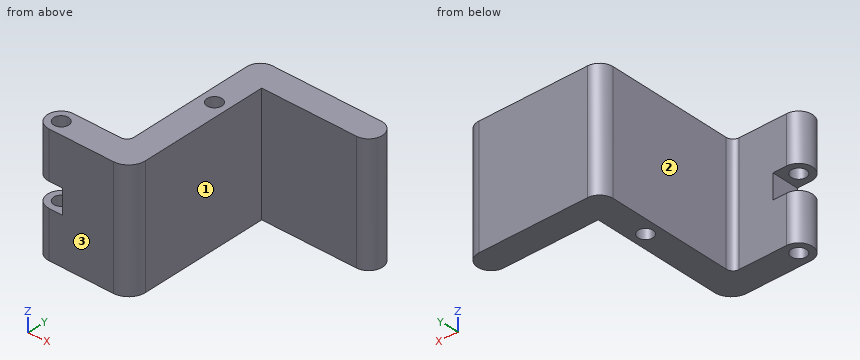
from build123d import *

# Parameters (mm, degrees)
BOSS_EXTRUDE1_DEPTH     = 87.5
SKETCH2_R               = 11
CUT_EXTRUDE1_DEPTH      = 175
FILLET1_R               = 10
FILLET2_R               = 25
CUT_EXTRUDE2_DEPTH      = 18
CUT_EXTRUDE2_DEPTH_BACK = 18
SKETCH3_W               = 40
SKETCH3_H               = 40
BOSS_EXTRUDE2_START     = -175
BOSS_EXTRUDE2_DEPTH     = 175


with BuildPart() as part:
    # Sketch1 → Boss-Extrude1 (new, symmetric)
    with BuildSketch(Plane.XY):
        with BuildLine():
            Line((-20, 20), (-20, 140))
            ThreePointArc((-20, 140), (0, 160), (20, 140))
            Line((20, 140), (20, -20))
            Line((20, -20), (-100, -20))
            ThreePointArc((-100, -20), (-120, 0), (-100, 20))
            Line((-100, 20), (-20, 20))
        make_face()
    extrude(amount=BOSS_EXTRUDE1_DEPTH, both=True)

    # Sketch2 → Cut-Extrude1 (cut)
    with BuildSketch(Plane.XY.offset(87.5)):
        with Locations((-100, 0)):
            Circle(SKETCH2_R)
        with Locations((0, 140)):
            Circle(SKETCH2_R)
    extrude(amount=-CUT_EXTRUDE1_DEPTH, mode=Mode.SUBTRACT)

    # Fillet1
    fillet1_edges = [part.edges().sort_by_distance(p)[0] for p in [
        (-20, 20, 0),
    ]]
    fillet(fillet1_edges, radius=FILLET1_R)

    # Fillet2
    fillet2_edges = [part.edges().sort_by_distance(p)[0] for p in [
        (20, -20, 0),
    ]]
    fillet(fillet2_edges, radius=FILLET2_R)

    # Sketch3 → Cut-Extrude2 (cut, two sides: drawn at the far end of the back side and taken through both)
    with BuildSketch(Plane.XY.offset(-CUT_EXTRUDE2_DEPTH_BACK)):
        with Locations((-100, 0)):
            Rectangle(SKETCH3_W, SKETCH3_H)
    extrude(amount=CUT_EXTRUDE2_DEPTH + CUT_EXTRUDE2_DEPTH_BACK, mode=Mode.SUBTRACT)

    # Sketch4 → Boss-Extrude2 (add)
    with BuildSketch(Plane(origin=(0, 0, -87.5), x_dir=(-1, 0, 0), z_dir=(0, 0, -1)).offset(BOSS_EXTRUDE2_START)):
        with BuildLine():
            ThreePointArc((-20, 140), (0, 160), (20, 140))
            Line((20, 140), (20, 215.09))
            ThreePointArc((20, 215.09), (14.142135624, 229.232135624), (0, 235.09))
            Line((0, 235.09), (-160, 235.09))
            ThreePointArc((-160, 235.09), (-180, 215.09), (-160, 195.09))
            Line((-160, 195.09), (-20, 195.09))
            Line((-20, 195.09), (-20, 140))
        make_face()
    extrude(amount=BOSS_EXTRUDE2_DEPTH)


solid = part.part
Could you check a few things on this model? Use its own coordinates, in mm. Face numbers are marked on the shaded views. A direction names the side the tool comes from. Coordinates: 2 decimals unless noted, no trailing zeros. Order: outer loops, then holes, each group sorted by start corner. A loop starts at its lowest first (then second) coordinate and runs counter-clockwise, first axis right, second up. Notation, with made-up numbers: (69, 48.25) - (108, 48.25) arc R26 ccw to (108, 65.25) - close; hole circle Ø9 at (80.5, 75.25). An arc over 180 degrees is marked (long way). Answer in a Markdown table with one row per item. Add a question column.
(1) If we section it at D-D, the plane x = 45.5: Please give me the cut outline in (y, z), then the cut area to 3 significant figures.
(2) On a 3-axis mill with a long thin cutter (end or side, diameter ignored), from which of +Z, -Z, +X, -X, +Y, -Y can I reach the whole of each face in a straight line? I mean the marked faces 1, 2 and 3. Say none if no direction works.
(3) If we section it at C-C, the plane z = 36: Please give me the cut outline in (x, y), then the cut area to 3 significant figures.
(4) If we section it at B-B, the plane z = -1: Please give me the cut outline in (x, y).
(5) Will these pins go through, and if not, where does the flat tip stop? pin 1 (1.5 mm diameter, centred on x = 22.5, y = 14.5, fed in from -Z); pin 2 (8 mm diameter, centred on y = 199, z = 59, fed in from -X); pin 3 (6 mm diameter, centred on y = 38, z = 10, fed in from +X); pin 4 (1 mm diameter, centred on x = -8.5, z = 2.5, fed in from +Y).
(6) I need wall thicknesses on L1, parallel to Y at x = -100, z = 45; L2, parallel to X at y = 176, z = 21; L3, parallel to X at y = 18.5, z = -4. Which ranges of each line are inside material? Lowest first, please.
(7) If we section it at A-A, the plane y = 140: Please give me the cut outline in (x, z), then the cut area to 3 significant figures.
Results are:
| question | item | result |
|---|---|---|
| 1 | outline | (195.09, -87.5) - (235.09, -87.5) - (235.09, 87.5) - (195.09, 87.5) - close |
| 1 | area | 7,000 mm2 |
| 2 | face 1 | +Z, -Z, +X, -Y |
| 2 | face 2 | +Z, -Z, -X, +Y |
| 2 | face 3 | +Z, -Z, +X, -X, -Y |
| 3 | outline | (-100, -20) - (-5, -20) arc R25 ccw to (20, 5) - (20, 195.09) - (160, 195.09) arc R20 ccw to (160, 235.09) - (0, 235.09) arc R20 ccw to (-20, 215.09) - (-20, 30) arc R10 cw to (-30, 20) - (-100, 20) arc R20 ccw to start; hole circle Ø22 at (-100, 0); hole circle Ø22 at (0, 140) |
| 3 | area | 19,300 mm2 |
| 4 | outline | (-80, -20) - (-5, -20) arc R25 ccw to (20, 5) - (20, 195.09) - (160, 195.09) arc R20 ccw to (160, 235.09) - (0, 235.09) arc R20 ccw to (-20, 215.09) - (-20, 30) arc R10 cw to (-30, 20) - (-80, 20) - close; hole circle Ø22 at (0, 140) |
| 5 | pin 1 | passes through |
| 5 | pin 2 | stops at x = -20 |
| 5 | pin 3 | stops at x = 20 |
| 5 | pin 4 | stops at y = 233.42 |
| 6 | L1 | y = -20 to -11, 11 to 20 |
| 6 | L2 | x = -20 to 20 |
| 6 | L3 | x = -80 to 20 |
| 7 | outline | (-20, -87.5) - (-11, -87.5) - (-11, 87.5) - (-20, 87.5) - close; (11, -87.5) - (20, -87.5) - (20, 87.5) - (11, 87.5) - close |
| 7 | area | 3,150 mm2 |
